Read the model definition and answer for the solid it produces. Units are mm, in the model's axes. Face numbers are marked on the shaded views. Coordinates: 2 decimals unless noted, no trailing zeros. Loops run counter-clockwise (first coordinate to the right, second up) from the corner with the lowest first, then second, coordinate; pieces in that order, holes last. Notation, with made-up numbers: (-31, 53.25) - (-2, 53.25) arc R8 cw to (-2, 59.25) - close; hole circle Ø11 at (53, 21). An arc over 180 degrees is marked (long way). Use one line per item in the form item = value. Start each with the question number.
1) A cutting plane is placed at C-C (z = -0.6). Give the vertices of the cut face in (x, y).
2) A cutting plane is placed at D-D (x = 23). Give the vertices of the cut face in (y, z).
3) The mould has two halves that part along X. Classify the marked faces 1, 2, 3 and 4: released by +X, released by -X, zero draft, split by the parting line, or undercut.
4) Consider line 1 (Y direction, x = 0, z = -2.95); line 2 (Y direction, x = 23, z = -0.2); line 3 (Y direction, x = -22, z = -0.55). Determine where each line is inside the solid, lowest interval first.
5) A cutting plane is placed at B-B (y = -22). Give the vertices of the cut face in (x, z), and give its area (3 significant figures).
6) Each of these flat-tipped pins is pushed along its axis until it touches: P1, Ø8, axis at x = -23, y = 1, coming from the +Z side; P2, Ø9.5, axis at x = 0, y = 24, coming from the +Z side; P3, Ø1.5, axis at x = 1.5, z = -0.5, coming from the -Y side. Where does it stop, or does it pass through?
7) A cutting plane is placed at A-A (x = 0). Give the vertices of the cut face in (y, z).
from build123d import *

# Parameters (mm, degrees)
F0_R           = 30
F1_DEPTH       = 4
F3_D           = 13.2
F3_DEPTH       = 12
F3_CSINK_D     = 26.88
F3_CSINK_ANGLE = 90
F3_TIP         = 3.9656800856
F5_D           = 6
F5_DEPTH       = 12
F5_CSINK_D     = 10
F5_CSINK_ANGLE = 90
F5_TIP         = 1.8025818571


with BuildPart() as f1:
    # F0 (on Top) → F1 (new body)
    with BuildSketch(Plane.XY):
        Circle(F0_R)
    extrude(amount=-F1_DEPTH)

    # F3
    with Locations(Plane.XY):
        with Locations((0, 0)):
            CounterSinkHole(F3_D / 2, F3_CSINK_D / 2, depth=F3_DEPTH, counter_sink_angle=F3_CSINK_ANGLE)
            with Locations((0, 0, -(F3_DEPTH + F3_TIP / 2))):  # 118° drill point
                Cone(0, F3_D / 2, F3_TIP, mode=Mode.SUBTRACT)

    # F5
    with Locations(Plane.XY):
        with Locations((-23, 1), (0, 24), (23, 1), (0, -22)):
            CounterSinkHole(F5_D / 2, F5_CSINK_D / 2, depth=F5_DEPTH, counter_sink_angle=F5_CSINK_ANGLE)
            with Locations((0, 0, -(F5_DEPTH + F5_TIP / 2))):  # 118° drill point
                Cone(0, F5_D / 2, F5_TIP, mode=Mode.SUBTRACT)


solid = f1.part
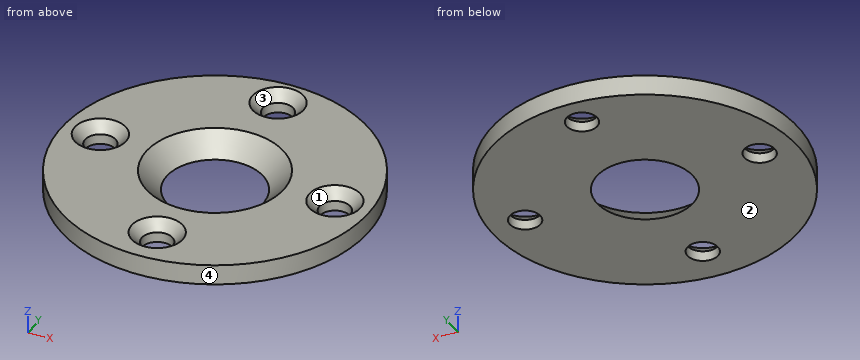
Found:
q1.outline = circle Ø60 at (0, 0); hole circle Ø8.8 at (-23, 1); hole circle Ø25.68 at (0, 0); hole circle Ø8.8 at (0, -22); hole circle Ø8.8 at (0, 24); hole circle Ø8.8 at (23, 1)
q2.outline = (-19.26, -4) - (-2, -4) - (-2, -2) - (-4, 0) - (-19.26, 0) - close; (4, -4) - (19.26, -4) - (19.26, 0) - (6, 0) - (4, -2) - close
q3.face_1 = undercut
q3.face_2 = zero draft
q3.face_3 = undercut
q3.face_4 = split by the parting line
q4.line_1 = -30 to -25, -19 to -10.49, 10.49 to 21, 27 to 30
q4.line_2 = -19.26 to -3.8, 5.8 to 19.26
q4.line_3 = -20.4 to -3.34, 5.34 to 20.4
q5.outline = (-20.4, -4) - (-3, -4) - (-3, -2) - (-5, 0) - (-20.4, 0) - close; (3, -4) - (20.4, -4) - (20.4, 0) - (5, 0) - (3, -2) - close
q5.area = 135 mm^2
q6.P1 = -1
q6.P2 = -0.25
q6.P3 = -29.99
q7.outline = (-30, -4) - (-25, -4) - (-25, -2) - (-27, 0) - (-30, 0) - close; (-19, -4) - (-9.44, -4) - (-13.44, 0) - (-17, 0) - (-19, -2) - close; (9.44, -4) - (21, -4) - (21, -2) - (19, 0) - (13.44, 0) - close; (27, -4) - (30, -4) - (30, 0) - (29, 0) - (27, -2) - close
